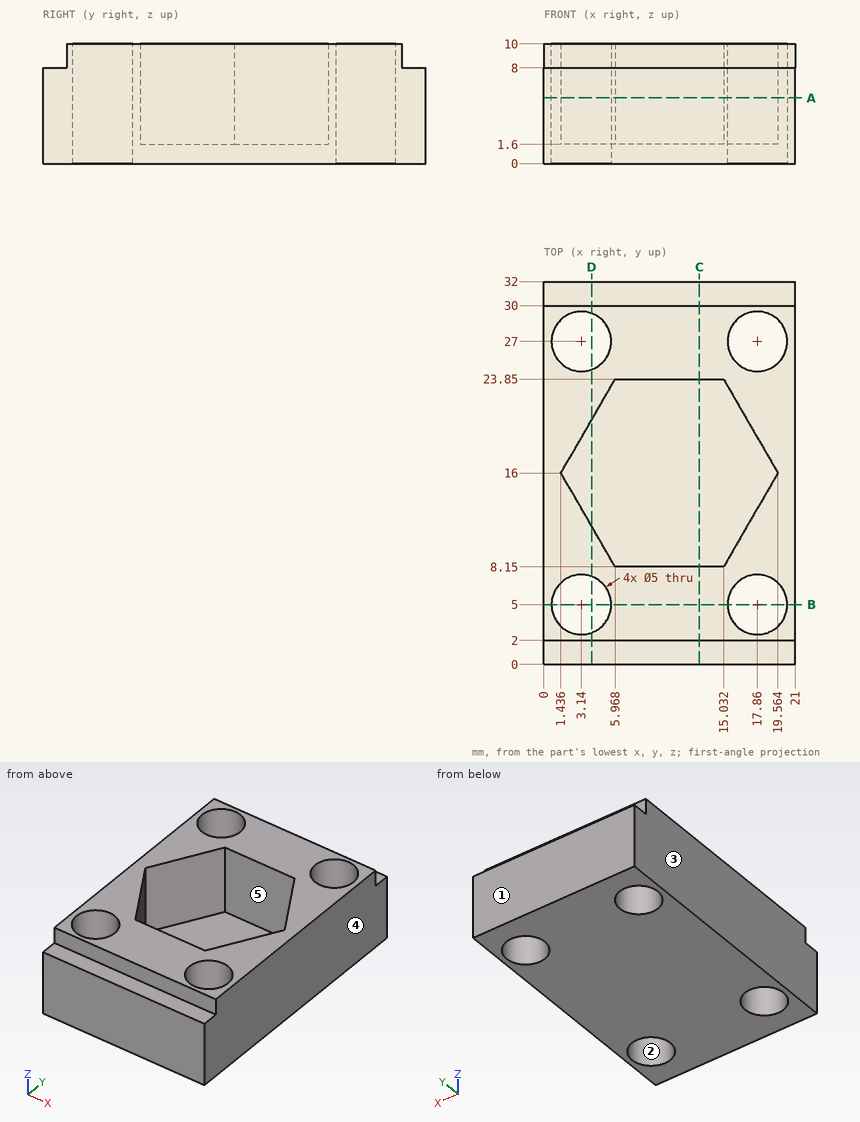
Can you work these out from the drawing? Everything is in mm from the part's minimum corner. A direction names the side the tool comes from. Coordinates: 2 decimals unless noted, no trailing zeros. Loops run counter-clockwise (first coordinate to the right, second up) from the corner with the lowest first, then second, coordinate; pieces in that order, holes last.
1) Imagine slicing it at A-A on z = 5.5. State how many separate pieces and enclosed holes the cut face has, plus the area to 3 significant figures.
2) Thinking about a two-plate mould opening in X: for the marked faces 1, 2 and 3, which applies, pulls with the +X half, pulls with the -X half, needs draft (parallel to the pull), parting line crosses it, or undercut?
3) Which directions (+Z, -Z, +X, -X, +Y, -Y) give clear straight access to the entire face, cutting with the end or side of a thin tool? Please do the marked faces 4 and 5.
4) Imagine slicing it at C-C on x = 13. List the corners of the cut face in (y, z) for me, plus the area to 3 significant figures.
5) Imagine slicing it at D-D on x = 4. List the corners of the cut face in (y, z) for me.
6) Imagine slicing it at B-B on y = 5. List the corners of the cut face in (x, z) for me, plus the area to 3 significant figures.
7) For pin 1 (1 mm diameter, centred on x = 17, z = 9, fed in from -Y); pin 2 (2 mm diameter, centred on x = 6, z = 9.5, fed in from +Y); pin 3 (2 mm diameter, centred on x = 14, y = 10, fed in from +Z), each with a flat end and sliding along its axis, tell me the tip position at first contact or that it passes through.
8) I need wall thicknesses on probe 1 along Y at (x, z) = (6, 9.25); probe 2 along Y at (x, z) = (3, 1) (1 decimal); probe 3 along Y at (x, z) = (18.5, 1). Which ranges of each line are inside material? Lowest first, please.
Completed:
1. separate pieces: 1
1. enclosed holes: 5
1. area: 380 mm2
2. face 1: needs draft
2. face 2: undercut
2. face 3: pulls with the -X half
3. face 4: +Z, -Z, +X, +Y, -Y
3. face 5: +Z
4. outline: (0, 0) - (32, 0) - (32, 8) - (30, 8) - (30, 10) - (23.85, 10) - (23.85, 1.6) - (8.15, 1.6) - (8.15, 10) - (2, 10) - (2, 8) - (0, 8) - close
4. area: 180 mm2
5. outline: (0, 0) - (2.65, 0) - (2.65, 10) - (2, 10) - (2, 8) - (0, 8) - close; (7.35, 0) - (24.65, 0) - (24.65, 10) - (20.44, 10) - (20.44, 1.6) - (11.56, 1.6) - (11.56, 10) - (7.35, 10) - close; (29.35, 0) - (32, 0) - (32, 8) - (30, 8) - (30, 10) - (29.35, 10) - close
6. outline: (0, 0) - (0.64, 0) - (0.64, 10) - (0, 10) - close; (5.64, 0) - (15.36, 0) - (15.36, 10) - (5.64, 10) - close; (20.36, 0) - (21, 0) - (21, 10) - (20.36, 10) - close
6. area: 110 mm2
7. pin 1: stops at y = 2
7. pin 2: stops at y = 30
7. pin 3: stops at z = 1.6
8. probe 1: y = 2 to 8.15, 23.85 to 30
8. probe 2: y = 0 to 2.5, 7.5 to 24.5, 29.5 to 32
8. probe 3: y = 0 to 2.58, 7.42 to 24.58, 29.42 to 32
